For this review, take the finished solid that the model builds, in its own axes (mm). A direction names the side the tool comes from. Round coordinates to 2 decimals unless told otherwise and drop trailing zeros. Use a Markdown table: item, result.
from build123d import *

# Parameters (mm, degrees)
F0_W     = 64.6
F0_H     = 68
F1_DEPTH = 20
F3_DEPTH = 6


with BuildPart() as f1:
    # F0 (on Top) → F1 (new body)
    with BuildSketch(Plane.XY):
        with Locations((19.1144577392, 24)):
            Rectangle(F0_W, F0_H)
    extrude(amount=F1_DEPTH)

    # F2 (on face) → F3 (cut)
    with BuildSketch(Plane(origin=(0, 0, 0), x_dir=(1, 0, 0), z_dir=(0, 0, -1))):
        with BuildLine():
            ThreePointArc((48.4144577392, 8), (47.707350958, 7.7071067812), (47.4144577392, 7))
            Line((47.4144577392, 7), (48.4144577392, 7))
            Line((48.4144577392, 7), (48.4144577392, 8))
        make_face()
        with BuildLine():
            ThreePointArc((49.1215645203, 7.7071067812), (48.7971411715, 7.9238795325), (48.4144577392, 8))
            Line((48.4144577392, 8), (48.4144577392, 7))
            Line((48.4144577392, 7), (49.1215645203, 7.7071067812))
        make_face()
        with BuildLine():
            Line((49.1215645203, 7.7071067812), (48.4144577392, 7))
            Line((48.4144577392, 7), (49.4144577392, 7))
            ThreePointArc((49.4144577392, 7), (49.3383372717, 7.3826834324), (49.1215645203, 7.7071067812))
        make_face()
        with BuildLine():
            ThreePointArc((49.4144577392, -55), (49.1215645203, -54.2928932188), (48.4144577392, -54))
            Line((48.4144577392, -54), (48.4144577392, -55))
            Line((48.4144577392, -55), (49.4144577392, -55))
        make_face()
        with BuildLine():
            ThreePointArc((49.1215645203, -55.7071067812), (49.3383372717, -55.3826834324), (49.4144577392, -55))
            Line((49.4144577392, -55), (48.4144577392, -55))
            Line((48.4144577392, -55), (49.1215645203, -55.7071067812))
        make_face()
        with BuildLine():
            Line((48.4144577392, -55), (48.4144577392, -56))
            ThreePointArc((48.4144577392, -56), (48.7971411715, -55.9238795325), (49.1215645203, -55.7071067812))
            Line((49.1215645203, -55.7071067812), (48.4144577392, -55))
        make_face()
        with BuildLine():
            Line((-10.1855422608, 7), (-9.1855422608, 7))
            ThreePointArc((-9.1855422608, 7), (-9.4784354797, 7.7071067812), (-10.1855422608, 8))
            Line((-10.1855422608, 8), (-10.1855422608, 7))
        make_face()
        with BuildLine():
            Line((-10.1855422608, 7), (-10.1855422608, 8))
            ThreePointArc((-10.1855422608, 8), (-10.5682256932, 7.9238795325), (-10.892649042, 7.7071067812))
            Line((-10.892649042, 7.7071067812), (-10.1855422608, 7))
        make_face()
        with BuildLine():
            Line((-11.1855422608, 7), (-10.1855422608, 7))
            Line((-10.1855422608, 7), (-10.892649042, 7.7071067812))
            ThreePointArc((-10.892649042, 7.7071067812), (-11.1094217934, 7.3826834324), (-11.1855422608, 7))
        make_face()
        with BuildLine():
            ThreePointArc((-10.1855422608, -56), (-9.4784354797, -55.7071067812), (-9.1855422608, -55))
            Line((-9.1855422608, -55), (-10.1855422608, -55))
            Line((-10.1855422608, -55), (-10.1855422608, -56))
        make_face()
        with BuildLine():
            Line((-10.1855422608, -56), (-10.1855422608, -55))
            Line((-10.1855422608, -55), (-10.892649042, -55.7071067812))
            ThreePointArc((-10.892649042, -55.7071067812), (-10.5682256932, -55.9238795325), (-10.1855422608, -56))
        make_face()
        with BuildLine():
            Line((-10.1855422608, -55), (-11.1855422608, -55))
            ThreePointArc((-11.1855422608, -55), (-11.1094217934, -55.3826834324), (-10.892649042, -55.7071067812))
            Line((-10.892649042, -55.7071067812), (-10.1855422608, -55))
        make_face()
    extrude(amount=-F3_DEPTH, mode=Mode.SUBTRACT)


solid = f1.part
Q1. Draft analysis for pull direction X (two halves, no side actions). For faces 1 (the flat face through (51.414, 24, 10)), 2 (the flat face through (19, 24, 0)), 3 (the flat face through (-10, -7, 3)), state which applies: pulls with the +X half, pulls with the -X half, needs draft (parallel to the pull), parting line crosses it, or undercut.
Determined:
| item | result |
|---|---|
| face 1 | pulls with the +X half |
| face 2 | needs draft |
| face 3 | undercut |
Q2. Machinability: for faces 4 (the flat face through (19, 24, 20)), 5 (the flat face through (-10, 55, 3)), which of the approach directions +Z, -Z, +X, -X, +Y, -Y give a long, thin tool a straight path to every point of the face, cutting with its end or side? Answer none if there is none.
Determined:
| item | result |
|---|---|
| face 4 | +Z, +X, -X, +Y, -Y |
| face 5 | -Z |
Q3. Clearance check with a flat-ended pin moving along its axis: pin 1 (0.8 mm diameter, centred on x = -10, y = 55.5, fed in from -Z). State where the tip first meets the part, or that it passes through.
Determined:
| item | result |
|---|---|
| pin 1 | stops at z = 6 |
